CAD build for the part. Positions are in the model's coordinates, mm. Face numbers are marked on the shaded views. A direction names the side the tool comes from. Give positions to 0.01 mm unless a question says otherwise; leave off trailing zeros. Loops run counter-clockwise (first coordinate to the right, second up) from the corner with the lowest first, then second, coordinate; pieces in that order, holes last.
Item 1: Probe probe 1 along Y at (x, z) = (0, 23) (3 decimals); probe 2 along Z at (x, y) = (19, -3); probe 3 along X at (y, z) = (-3.5, 14.5). List the from-to ranges inside material, lowest first.
Item 2: Saw through at A-A on x = 0. Give the cut face in (y, z) (3 decimals).
Item 3: Mould opens along Y. For the marked faces 3, 4, 5 and 6 say: released by +Y, released by -Y, zero draft, split by the parting line, or undercut.
Item 4: Saw through at B-B on y = 0. Give the cut face in (x, z), plus the area to 3 significant figures.
Item 5: Drop flat-ended pins along their axis: P1, Ø1.5, axis at x = 1, z = 11.5, coming from the -Y side; P2, Ø12.5, axis at y = -2.5, z = 24, coming from the +X side; P3, Ø10, axis at x = 9, z = 6, coming from the -Y side. Give the stop position or say it passes through.
Item 6: Which spindle directions (+Z, -Z, +X, -X, +Y, -Y) get a long thin tool onto all of the face, cutting with end or side? Do the marked faces 1 and 2. Say none if no direction does.
Item 7: Saw through at C-C on z = 15. Give the cut face in (x, y) (3 decimals).
Item 8: Saw through at D-D on y = -10. Give the cut face in (x, z).
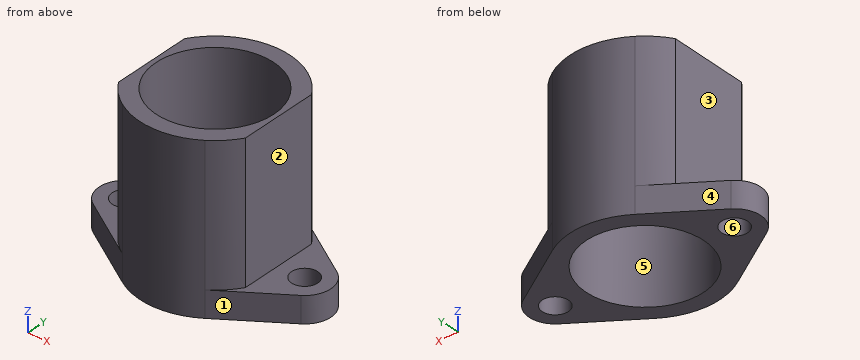
from build123d import *

# Parameters (mm, degrees)
F0_R     = 11.43
F0_R_2   = 2.54
F2_DEPTH = 5.08
F1_R     = 11.43
F3_DEPTH = 31.75


with BuildPart() as f2:
    # F0 (on Top) → F2 (new body)
    with BuildSketch(Plane.XY):
        with BuildLine():
            Line((12.319, 0), (12.319, 7.84527))
            ThreePointArc((12.319, 7.84527), (10.390293, 10.263909), (7.995438, 12.22207))
            ThreePointArc((7.995438, 12.22207), (0, 14.605), (-7.995438, 12.22207))
            ThreePointArc((-7.995438, 12.22207), (-10.390293, 10.263909), (-12.319, 7.84527))
            Line((-12.319, 7.84527), (-12.319, 0))
            Line((-12.319, 0), (-12.319, -7.84527))
            ThreePointArc((-12.319, -7.84527), (-10.390293, -10.263909), (-7.995438, -12.22207))
            ThreePointArc((-7.995438, -12.22207), (0, -14.605), (7.995438, -12.22207))
            ThreePointArc((7.995438, -12.22207), (10.390293, -10.263909), (12.319, -7.84527))
            Line((12.319, -7.84527), (12.319, 0))
        make_face()
        Circle(F0_R, mode=Mode.SUBTRACT)
        with BuildLine():
            ThreePointArc((7.995438, 12.22207), (10.390293, 10.263909), (12.319, 7.84527))
            Line((12.319, 7.84527), (12.319, 0))
            Line((12.319, 0), (12.319, -7.84527))
            ThreePointArc((12.319, -7.84527), (10.390293, -10.263909), (7.995438, -12.22207))
            Line((7.995438, -12.22207), (20.180022, -4.251155))
            ThreePointArc((20.180022, -4.251155), (22.479, 0), (20.180022, 4.251155))
            Line((20.180022, 4.251155), (7.995438, 12.22207))
        make_face()
        with Locations((17.399, 0)):
            Circle(F0_R_2, mode=Mode.SUBTRACT)
        with BuildLine():
            ThreePointArc((-12.319, 7.84527), (-10.390293, 10.263909), (-7.995438, 12.22207))
            Line((-7.995438, 12.22207), (-20.180022, 4.251155))
            ThreePointArc((-20.180022, 4.251155), (-22.479, 0), (-20.180022, -4.251155))
            Line((-20.180022, -4.251155), (-7.995438, -12.22207))
            ThreePointArc((-7.995438, -12.22207), (-10.390293, -10.263909), (-12.319, -7.84527))
            Line((-12.319, -7.84527), (-12.319, 0))
            Line((-12.319, 0), (-12.319, 7.84527))
        make_face()
        with Locations((-17.399, 0)):
            Circle(F0_R_2, mode=Mode.SUBTRACT)
    extrude(amount=F2_DEPTH)

    # F1 (on face) → F3 (join)
    with BuildSketch(Plane.XY):
        with BuildLine():
            Line((12.319, -7.84527), (12.319, 0))
            Line((12.319, 0), (12.319, 7.84527))
            ThreePointArc((12.319, 7.84527), (10.390293, 10.263909), (7.995438, 12.22207))
            ThreePointArc((7.995438, 12.22207), (0, 14.605), (-7.995438, 12.22207))
            ThreePointArc((-7.995438, 12.22207), (-10.390293, 10.263909), (-12.319, 7.84527))
            Line((-12.319, 7.84527), (-12.319, 0))
            Line((-12.319, 0), (-12.319, -7.84527))
            ThreePointArc((-12.319, -7.84527), (-10.390293, -10.263909), (-7.995438, -12.22207))
            ThreePointArc((-7.995438, -12.22207), (0, -14.605), (7.995438, -12.22207))
            ThreePointArc((7.995438, -12.22207), (10.390293, -10.263909), (12.319, -7.84527))
        make_face()
        Circle(F1_R, mode=Mode.SUBTRACT)
    extrude(amount=F3_DEPTH)


solid = f2.part
Results below:
1. probe 1: y = -14.605 to -11.43, 11.43 to 14.605
1. probe 2: z = 0 to 5.08
1. probe 3: x = -12.32 to -10.88, 10.88 to 12.32
2. outline: (-14.605, 0) - (-11.43, 0) - (-11.43, 31.75) - (-14.605, 31.75) - close; (11.43, 0) - (14.605, 0) - (14.605, 31.75) - (11.43, 31.75) - close
3. face 3: zero draft
3. face 4: released by +Y
3. face 5: undercut
3. face 6: undercut
4. outline: (-22.48, 0) - (-19.94, 0) - (-19.94, 5.08) - (-22.48, 5.08) - close; (-14.86, 0) - (-11.43, 0) - (-11.43, 31.75) - (-12.32, 31.75) - (-12.32, 5.08) - (-14.86, 5.08) - close; (11.43, 0) - (14.86, 0) - (14.86, 5.08) - (12.32, 5.08) - (12.32, 31.75) - (11.43, 31.75) - close; (19.94, 0) - (22.48, 0) - (22.48, 5.08) - (19.94, 5.08) - close
4. area: 108 mm2
5. P1: stops at y = -14.6
5. P2: stops at x = 12.32
5. P3: stops at y = -14.05
6. face 1: +Z, -Z, +X, -Y
6. face 2: +Z, +X, +Y, -Y
7. outline: (-12.319, -7.845) arc R14.605 ccw to (-7.995, -12.222) arc R14.605 ccw to (7.995, -12.222) arc R14.605 ccw to (12.319, -7.845) - (12.319, 7.845) arc R14.605 ccw to (7.995, 12.222) arc R14.605 ccw to (-7.995, 12.222) arc R14.605 ccw to (-12.319, 7.845) - close; hole circle Ø22.86 at (0, 0)
8. outline: (-11.39, 0) - (-5.54, 0) - (-5.54, 31.75) - (-10.64, 31.75) - (-10.64, 5.08) - (-11.39, 5.08) - close; (5.54, 0) - (11.39, 0) - (11.39, 5.08) - (10.64, 5.08) - (10.64, 31.75) - (5.54, 31.75) - close
